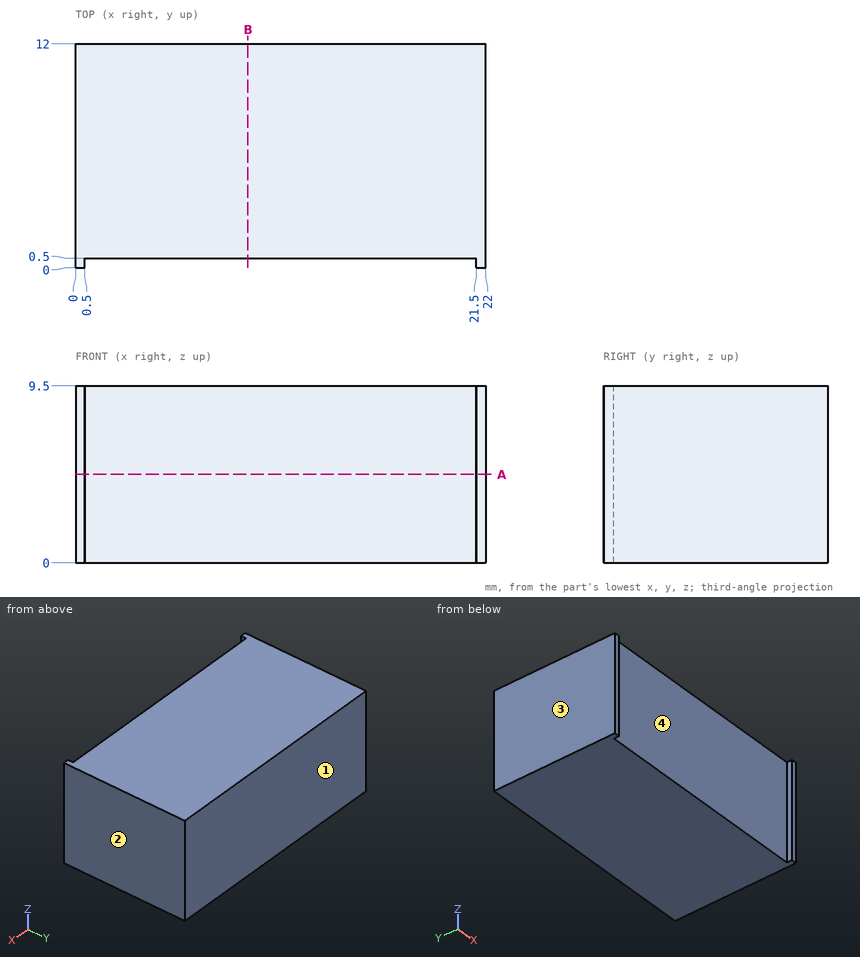
Job drawing, mm, ordinate dimensions from the low corner. One solid piece. Round coordinates to 2 decimals unless told otherwise and drop trailing zeros. Order: outer loops, then holes, each group sorted by start corner. A loop starts at its lowest first (then second) coordinate and runs counter-clockwise, first axis right, second up. Notation, with made-up numbers: M -12.5,-37 L 37.5,-37 A25 cw 37.5,-10 Z; hole C 1,81.25 d1. An arc over 180 degrees is marked long. Write each question's results on one line, items separated by ' | '. Start each with the question number.
(1) Two-plate mould, pull along X, no slides. Class the marked faces 1, 2, 3 and 4: pulls with the +X half, pulls with the -X half, needs draft (parallel to the pull), parting line crosses it, or undercut.
(2) Probe probe 1 along Y at (x, z) = (9.75, 1.75). List the from-to ranges inside material, lowest first. Write a range as from..to.
(3) Saw through at B-B, the plane x = 9.25. Give the cut face in (y, z).
(4) Saw through at A-A, the plane z = 4.75. Give the cut face in (x, y), then the cut area to 4 significant figures.
(5) Drop a flat-ended pin along its axis: pin 1 (5 mm diameter, centred on x = 15, z = 2.5, fed in from -Y). Give the stop position or say it passes through.
Established:
1) face 1: needs draft | face 2: pulls with the +X half | face 3: pulls with the -X half | face 4: undercut
2) probe 1: y = 0.5..12
3) outline: M 0.5,0 L 12,0 L 12,9.5 L 0.5,9.5 Z
4) outline: M 0,0 L 0.5,0 L 0.5,0.5 L 21.5,0.5 L 21.5,0 L 22,0 L 22,12 L 0,12 Z | area: 253.5 mm^2
5) pin 1: stops at y = 0.5
